Here's how the part is built. I have some questions about the finished solid (model axes, mm). A direction names the side the tool comes from. Give positions to 0.01 mm unless a question says otherwise; leave off trailing zeros. Write each loop counter-clockwise with the first axis right and the second up, starting at its lowest first coordinate (ties: lowest second). Pieces come first, ordered by that corner, then holes. Notation, with made-up numbers: M 3.5,89 L 39.5,89 A18 ccw 39.5,102 Z; hole C -21.75,46.5 d2. An arc over 180 degrees is marked long. Answer as CSV lines item,"result". Start each with the question number.
Q1. Suppose I cut it at C-C (y = 0). Write out the boundary of the cut face in (x, z).
Q2. For pin 1 (4 mm diameter, centred on x = -45, y = 63, fed in from -Z); pin 2 (16 mm diameter, centred on x = 0, y = 0, fed in from +Z); pin 3 (6 mm diameter, centred on x = -1, y = -4, fed in from -Z), each with a flat end and sliding along its axis, tell me the tip position at first contact or that it passes through.
Q3. If I drill on line 1 along X through (y, z) = (0, 7); line 2 along Y through (x, z) = (0, 9.75); line 3 along Z through (x, y) = (55, -43), over which ranges is the centre line in solid material (lowest first)?
Q4. Suppose I cut it at B-B (z = 162). Write out the boundary of the cut face in (x, y).
Q5. Thinking about a two-plate mould opening in X: for faces 5 (the cylindrical face through (101.58, 89.23, 187.15)), 6 (the cylindrical face through (1.32, 75.59, 43.01)), 7 (the flat face through (-104.588, 0, 23)), 8 (the flat face through (0, 0, 20)), which applies, +X half, -X half, draft (parallel to the pull), parting line (faces both ways), or undercut?
Q6. Suppose I cut it at A-A (x = 77). Write out the boundary of the cut face in (y, z).
Q7. On a 3-axis mill with a long thin cutter (end or side, diameter ignored), from which of +Z, -Z, +X, -X, +Y, -Y can I reach the whole of each face in a straight line? I mean faces 1 (the cylindrical face through (-2.17, 9.76, 9.86)), 2 (the cylindrical face through (101.58, 81.29, 115.91)), 3 (the cylindrical face through (-101.74, -9.67, 36.99)), 4 (the flat face through (-1, 78.439, 114)). Say none if no direction works.
Q8. Suppose I cut it at D-D (x = 0). Write out the boundary of the cut face in (y, z), then the cut area to 3 significant figures.
```python
from build123d import *

# Parameters (mm, degrees)
F0_W     = 209.176
F0_H     = 200
F1_DEPTH = 40
F2_W     = 209.176
F2_H     = 21.5614646673
F3_DEPTH = 150
F4_R     = 10
F5_DEPTH = 20
F6_F1_R  = 10
F6_F2_R  = 10
F7_R     = 10


with BuildPart() as f1:
    # F0 (on Top) → F1 (new body)
    with BuildSketch(Plane.XY):
        Rectangle(F0_W, F0_H)
    extrude(amount=F1_DEPTH)

    # F2 (on face) → F3 (join)
    with BuildSketch(Plane.XY.offset(40)):
        with Locations((0, 89.2192676663)):
            Rectangle(F2_W, F2_H)
    extrude(amount=F3_DEPTH)

    # F4 (on face) → F5 (cut)
    with BuildSketch(Plane(origin=(0, 0, 0), x_dir=(1, 0, 0), z_dir=(0, 0, -1))):
        Circle(F4_R)
    extrude(amount=-F5_DEPTH, mode=Mode.SUBTRACT)

    # F6: fillet of radius 10 on 10 edges, made by hand

    # F6_f1
    f6_f1_edges = [f1.edges().sort_by_distance(p)[0] for p in [
        (0, 78.4385353327, 40),
    ]]
    fillet(f6_f1_edges, radius=F6_F1_R)

    # F6_f2
    f6_f2_edges = [f1.edges().sort_by_distance(p)[0] for p in [
        (0, 78.4385353327, 190),
        (0, 100, 190),
        (-104.588, 89.2192676663, 190),
        (104.588, 89.2192676663, 190),
        (-104.588, 78.4385353327, 120),
        (104.588, 78.4385353327, 120),
        (104.588, 100, 95),
        (-104.588, 100, 95),
        (0, 100, 0),
        (104.588, 75.5096031445, 42.9289321881),
        (-104.588, 75.5096031445, 42.9289321881),
    ]]
    fillet(f6_f2_edges, radius=F6_F2_R)

    # F7
    f7_edges = [f1.edges().sort_by_distance(p)[0] for p in [
        (0, -100, 40),
    ]]
    fillet(f7_edges, radius=F7_R)


solid = f1.part
```
Resolved:
1,outline,"M -104.59,0 L -10,0 L -10,20 L 10,20 L 10,0 L 104.59,0 L 104.59,30 A10 ccw 94.59,40 L -94.59,40 A10 ccw -104.59,30 Z"
2,pin 1,"z = 0"
2,pin 2,"z = 40"
2,pin 3,"z = 20"
3,line 1,"-104.59 to -10, 10 to 104.59"
3,line 2,"-100 to -10, 10 to 100"
3,line 3,"0 to 40"
4,outline,"M -104.59,88.44 A10 ccw -94.59,78.44 L 94.59,78.44 A10 ccw 104.59,88.44 L 104.59,90 A10 ccw 94.59,100 L -94.59,100 A10 ccw -104.59,90 Z"
5,face 5,"+X half"
5,face 6,"draft"
5,face 7,"-X half"
5,face 8,"undercut"
6,outline,"M -100,0 L 90,0 A10 ccw 100,10 L 100,180 A10 ccw 90,190 L 88.44,190 A10 ccw 78.44,180 L 78.44,50 A10 cw 68.44,40 L -90,40 A10 ccw -100,30 Z"
7,face 1,"-Z"
7,face 2,"+Z, +X, -Y"
7,face 3,"+Z, -X, -Y"
7,face 4,"+Z, +X, -X, -Y"
8,outline,"M -100,0 L -10,0 L -10,20 L 10,20 L 10,0 L 90,0 A10 ccw 100,10 L 100,180 A10 ccw 90,190 L 88.44,190 A10 ccw 78.44,180 L 78.44,50 A10 cw 68.44,40 L -90,40 A10 ccw -100,30 Z"
8,area,"10,800 mm^2"
